Can you work these out from the drawing? Everything is in mm from the part's minimum corner. Coordinates: 2 decimals unless noted, no trailing zeros. Write each loop counter-clockwise with the first axis right and the second up, starting at its lowest first coordinate (ties: lowest second). Pieces come first, ordered by that corner, then holes. Notation, with made-up numbers: M 40,65.25 L 63,65.25 A24 cw 63,87.25 Z; hole C 86.5,16.5 d2. An arc over 180 degrees is marked long. Write item = value, one per line.
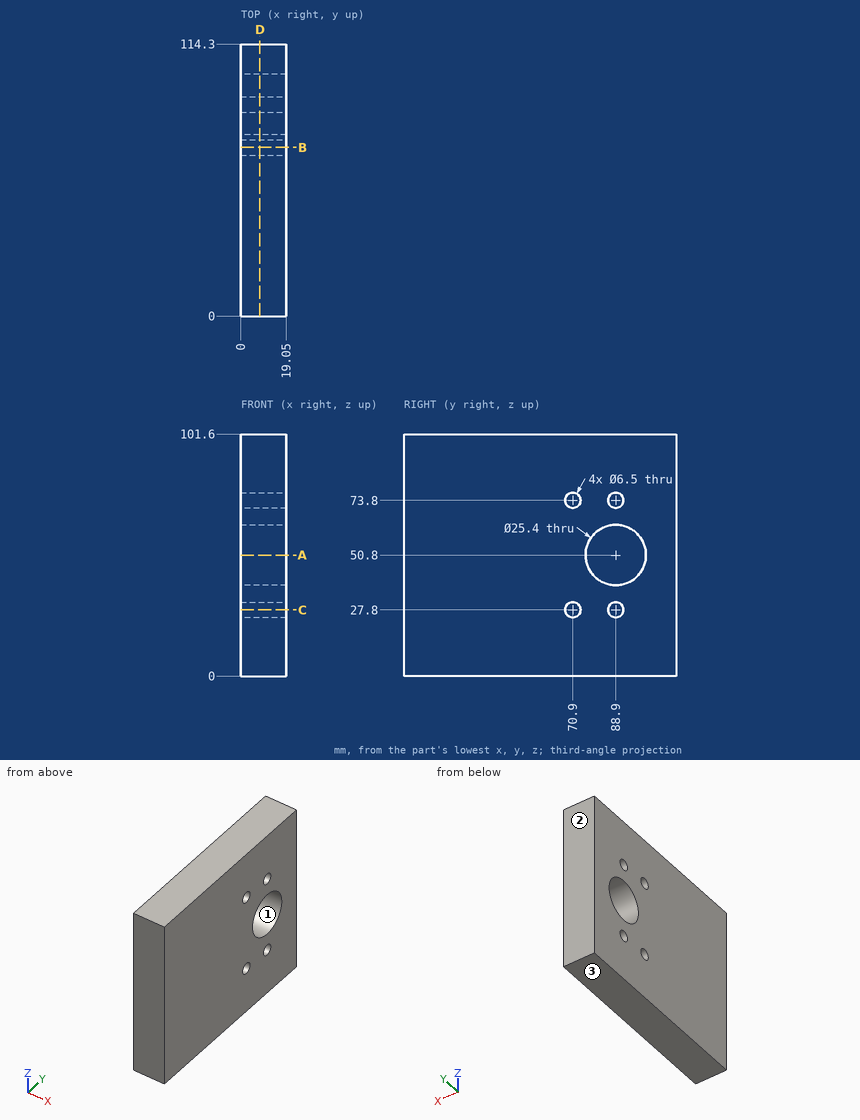
Item 1: Imagine slicing it at B-B (y = 70.9). Write out the boundary of the cut face in (x, z).
Numbers:
outline = M 0,0 L 19.05,0 L 19.05,24.55 L 0,24.55 Z; M 0,31.05 L 19.05,31.05 L 19.05,70.55 L 0,70.55 Z; M 0,77.05 L 19.05,77.05 L 19.05,101.6 L 0,101.6 Z
Item 2: Imagine slicing it at C-C (z = 27.8). Write out the boundary of the cut face in (x, y).
Numbers:
outline = M 0,0 L 19.05,0 L 19.05,67.65 L 0,67.65 Z; M 0,74.15 L 19.05,74.15 L 19.05,85.65 L 0,85.65 Z; M 0,92.15 L 19.05,92.15 L 19.05,114.3 L 0,114.3 Z
Item 3: I'm going to push a flat-ended pin straight in: P1, Ø6, axis at y = 88.9, z = 73.8, coming from the +X side. Where does the tip first touch, or does it pass through?
Numbers:
P1 = through
Item 4: Imagine slicing it at D-D (x = 8). Write out the boundary of the cut face in (y, z), and give its area (3 significant figures).
Numbers:
outline = M 0,0 L 114.3,0 L 114.3,101.6 L 0,101.6 Z; hole C 70.9,27.8 d6.5; hole C 70.9,73.8 d6.5; hole C 88.9,50.8 d25.4; hole C 88.9,27.8 d6.5; hole C 88.9,73.8 d6.5
area = 11,000 mm²
Item 5: If I drill on line 1 along Z through (x, y) = (10, 88.9); line 2 along Y through (x, z) = (11.75, 73.8); line 3 along Y through (x, z) = (4.75, 50.8), over which ranges is the centre line in solid material (lowest first)?
Numbers:
line_1 = 0 to 24.55, 31.05 to 38.1, 63.5 to 70.55, 77.05 to 101.6
line_2 = 0 to 67.65, 74.15 to 85.65, 92.15 to 114.3
line_3 = 0 to 76.2, 101.6 to 114.3
Item 6: Imagine slicing it at A-A (z = 50.8). Write out the boundary of the cut face in (x, y), and give its area (3 significant figures).
Numbers:
outline = M 0,0 L 19.05,0 L 19.05,76.2 L 0,76.2 Z; M 0,101.6 L 19.05,101.6 L 19.05,114.3 L 0,114.3 Z
area = 1,690 mm²
Item 7: If we mould it in two halves opening along Y, with no side actions, what happens to the marked faces 1, 2 and 3? For each: pulls with the +Y half, pulls with the -Y half, needs draft (parallel to the pull), parting line crosses it, or undercut.
Numbers:
face_1 = undercut
face_2 = pulls with the +Y half
face_3 = needs draft
